```python
from build123d import *

# Parameters (mm, degrees)
SKETCH_1_W               = 40
SKETCH_1_H               = 40
SKETCH_2_W               = 10
SKETCH_2_H               = 10
EXTRUDE_1_DEPTH          = 800
PATTERN_LINEAR_1_COUNT   = 7
PATTERN_LINEAR_1_PITCH   = 110
MIRROR_1_COPY_1_SKETCH_W = 10
MIRROR_1_COPY_1_SKETCH_H = 10
MIRROR_1_COPY_1_DEPTH    = 800
MIRROR_1_COPY_2_SKETCH_W = 10
MIRROR_1_COPY_2_SKETCH_H = 10
MIRROR_1_COPY_2_DEPTH    = 800
MIRROR_1_COPY_3_SKETCH_W = 10
MIRROR_1_COPY_3_SKETCH_H = 10
MIRROR_1_COPY_3_DEPTH    = 800
MIRROR_1_COPY_4_SKETCH_W = 10
MIRROR_1_COPY_4_SKETCH_H = 10
MIRROR_1_COPY_4_DEPTH    = 800
MIRROR_1_COPY_5_SKETCH_W = 10
MIRROR_1_COPY_5_SKETCH_H = 10
MIRROR_1_COPY_5_DEPTH    = 800
MIRROR_1_COPY_6_SKETCH_W = 10
MIRROR_1_COPY_6_SKETCH_H = 10
MIRROR_1_COPY_6_DEPTH    = 800


with BuildPart() as part:
    # По траектории1: sweep along a curve in space
    with BuildLine() as sweep_1_path:
        Line((0, 0, 0), (0, 840, 0))
        Line((0, 840, 0), (1650, 840, 0))
        Line((1650, 0, 0), (1650, 840, 0))
        Line((0, 0, 0), (1650, 0, 0))
    # Эскиз1 → По траектории1 (sweep)
    with BuildSketch(Plane(origin=(0, 0, 0), x_dir=(1, 0, 0), z_dir=(0, 1, 0))):
        Rectangle(SKETCH_1_W, SKETCH_1_H)
    sweep(path=sweep_1_path.line, transition=Transition.RIGHT)

    # Эскиз2 → Бобышка-Вытянуть1 (add)
    with BuildSketch(Plane(origin=(0, 20, 0), x_dir=(1, 0, 0), z_dir=(0, 1, 0))):
        with Locations((770, 0)):
            Rectangle(SKETCH_2_W, SKETCH_2_H)
    extrude_1 = extrude(amount=EXTRUDE_1_DEPTH)

    # Линейный массив1: Бобышка-Вытянуть1 ×7
    with Locations(*[(-i * PATTERN_LINEAR_1_PITCH, 0, 0) for i in range(1, PATTERN_LINEAR_1_COUNT)]):
        add(extrude_1)

    # Зеркальное отражение1: Бобышка-Вытянуть1 across plane
    add(extrude_1.mirror(Plane.ZY.offset(-825)))

    # Зеркальное отражение1 copy 1 sketch → Зеркальное отражение1 copy 1 (add)
    with BuildSketch(Plane(origin=(1760, 20, 0), x_dir=(-1, 0, 0), z_dir=(0, 1, 0))):
        with Locations((770, 0)):
            Rectangle(MIRROR_1_COPY_1_SKETCH_W, MIRROR_1_COPY_1_SKETCH_H)
    extrude(amount=MIRROR_1_COPY_1_DEPTH)

    # Зеркальное отражение1 copy 2 sketch → Зеркальное отражение1 copy 2 (add)
    with BuildSketch(Plane(origin=(1870, 20, 0), x_dir=(-1, 0, 0), z_dir=(0, 1, 0))):
        with Locations((770, 0)):
            Rectangle(MIRROR_1_COPY_2_SKETCH_W, MIRROR_1_COPY_2_SKETCH_H)
    extrude(amount=MIRROR_1_COPY_2_DEPTH)

    # Зеркальное отражение1 copy 3 sketch → Зеркальное отражение1 copy 3 (add)
    with BuildSketch(Plane(origin=(1980, 20, 0), x_dir=(-1, 0, 0), z_dir=(0, 1, 0))):
        with Locations((770, 0)):
            Rectangle(MIRROR_1_COPY_3_SKETCH_W, MIRROR_1_COPY_3_SKETCH_H)
    extrude(amount=MIRROR_1_COPY_3_DEPTH)

    # Зеркальное отражение1 copy 4 sketch → Зеркальное отражение1 copy 4 (add)
    with BuildSketch(Plane(origin=(2090, 20, 0), x_dir=(-1, 0, 0), z_dir=(0, 1, 0))):
        with Locations((770, 0)):
            Rectangle(MIRROR_1_COPY_4_SKETCH_W, MIRROR_1_COPY_4_SKETCH_H)
    extrude(amount=MIRROR_1_COPY_4_DEPTH)

    # Зеркальное отражение1 copy 5 sketch → Зеркальное отражение1 copy 5 (add)
    with BuildSketch(Plane(origin=(2200, 20, 0), x_dir=(-1, 0, 0), z_dir=(0, 1, 0))):
        with Locations((770, 0)):
            Rectangle(MIRROR_1_COPY_5_SKETCH_W, MIRROR_1_COPY_5_SKETCH_H)
    extrude(amount=MIRROR_1_COPY_5_DEPTH)

    # Зеркальное отражение1 copy 6 sketch → Зеркальное отражение1 copy 6 (add)
    with BuildSketch(Plane(origin=(2310, 20, 0), x_dir=(-1, 0, 0), z_dir=(0, 1, 0))):
        with Locations((770, 0)):
            Rectangle(MIRROR_1_COPY_6_SKETCH_W, MIRROR_1_COPY_6_SKETCH_H)
    extrude(amount=MIRROR_1_COPY_6_DEPTH)


solid = part.part
```
Work out the finished part from the listing and answer in its coordinate system (mm). A direction names the side the tool comes from. Round coordinates to 2 decimals unless told otherwise and drop trailing zeros. Loops run counter-clockwise (first coordinate to the right, second up) from the corner with the lowest first, then second, coordinate; pieces in that order, holes last. Notation, with made-up numbers: (71, 0.25) -> (83, 0.25) arc R6 cw to (83, 9.25) -> close; hole circle Ø9 at (-25, 23.25). An arc over 180 degrees is marked (long way). Write each question's results on one line, items separated by ' | '. Start each with the question number.
1. Given pin 1 Ø3 at (x, y) = (1431, 518) entering from +Z; pin 2 Ø5 at (x, y) = (442, 367) entering from -Z, each flat-ended and moving along its own axis, determine where each tip first touches the part or whether it passes through.
2. Section A-A (x = 1281.5) is taken. Determine the outline of the cut face in (y, z), plus the area to 3 significant figures.
3. Find the intervals of material crossed by probe 1 along X at (y, z) = (526, -7); probe 2 along Y at (x, z) = (1403, -11.5); probe 3 along Z at (x, y) = (107.5, 467), in increasing order. Write a range as from..to.
4. Section B-B (z = -13) is taken. Determine the outline of the cut face in (x, y), plus the area to 3 significant figures.
5. Section C-C (y = 387.5) is taken. State how many separate pieces and enclosed holes the cut face has, plus the area to 3 significant figures.
6. A tool of negligible diameter and unlimited length cuts with its end or side. For faces 4 (the face through (20, 426, 0)), 5 (the face through (758, -2, 20)), from which of +Z, -Z, +X, -X, +Y, -Y can it reach the whole face along a straight path? Write none if from no direction.
7. For a pull along X with two mould halves and no side action, classify faces 1 (the face through (1670, 414, 0)), 2 (the face through (892, -2, -20)), 3 (the face through (836, 820, 0)) as +X half, -X half, draft (parallel to the pull), parting line (faces both ways), or undercut.
Evaluation:
1) pin 1: stops at z = 5 | pin 2: stops at z = -5
2) outline: (-20, -20) -> (20, -20) -> (20, 20) -> (-20, 20) -> close; (820, -20) -> (860, -20) -> (860, 20) -> (820, 20) -> close | area: 3,200 mm2
3) probe 1: x = -20..20, 1630..1670 | probe 2: y = -20..20, 820..860 | probe 3: z = -5..5
4) outline: (-20, -20) -> (1670, -20) -> (1670, 860) -> (-20, 860) -> close; hole (20, 20) -> (1630, 20) -> (1630, 820) -> (20, 820) -> close | area: 199,000 mm2
5) separate pieces: 16 | enclosed holes: 0 | area: 4,600 mm2
6) face 4: +Z, -Z | face 5: +Z, +X, -X, +Y, -Y
7) face 1: +X half | face 2: draft | face 3: undercut
